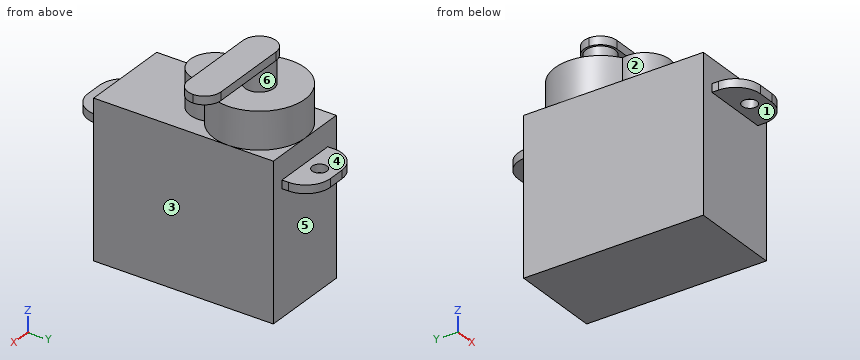
from build123d import *

# Parameters (mm, degrees)
F0_W      = 11
F0_H      = 21.8
F1_DEPTH  = 18.8
F3_W      = 8
F3_H      = 3.8
F3_R      = 0.9
F4_DEPTH  = 1
F6_DEPTH  = 4.5
F7_R      = 1.75
F8_DEPTH  = 3.5
F10_W     = 13.6
F10_H     = 4
F11_DEPTH = 1
F12_R     = 1.99999
F13_R     = 3


# Not quite as in the source:
# - a fillet or chamfer is up to 0.001 mm smaller than in the source, because OpenCascade refuses the exact size


with BuildPart() as f1:
    # F0 (on Top) → F1 (new body)
    with BuildSketch(Plane.XY):
        Rectangle(F0_W, F0_H)
    extrude(amount=F1_DEPTH)

    # F3 (on offset) → F4 (join)
    with BuildSketch(Plane.XY.offset(14.9)):
        with Locations((0, 12.8)):
            Rectangle(F3_W, F3_H)
        with Locations((0, 12.7)):
            Circle(F3_R, mode=Mode.SUBTRACT)
        with Locations((0, -12.8)):
            Rectangle(F3_W, F3_H)
        with Locations((0, -12.7)):
            Circle(F3_R, mode=Mode.SUBTRACT)
    extrude(amount=F4_DEPTH)

    # F5 (on face) → F6 (join)
    with BuildSketch(Plane.XY.offset(18.8)):
        with BuildLine():
            ThreePointArc((-2.9092231591, 0.7324074074), (0, -3), (2.9092231591, 0.7324074074))
            ThreePointArc((2.9092231591, 0.7324074074), (0, 10.9), (-2.9092231591, 0.7324074074))
        make_face()
    extrude(amount=F6_DEPTH)

    # F7 (on face) → F8 (join)
    with BuildSketch(Plane.XY.offset(23.3)):
        with Locations((0, 5.4)):
            Circle(F7_R)
    extrude(amount=F8_DEPTH)

    # F10 (on offset) → F11 (join)
    with BuildSketch(Plane(origin=(0, 0, 26.6), x_dir=(1, 0, 0), z_dir=(0, 0, -1))):
        with Locations((4.8, -5.4)):
            Rectangle(F10_W, F10_H)
    extrude(amount=-F11_DEPTH)

    # F12 (radius 2 in the source; OpenCascade refuses exactly that, so slightly less here)
    f12_edges = [f1.edges().sort_by_distance(p)[0] for p in [
        (11.6, 3.4, 27.1),
        (11.6, 7.4, 27.1),
        (-2, 7.4, 27.1),
        (-2, 3.4, 27.1),
    ]]
    fillet(f12_edges, radius=F12_R)

    # F13
    f13_edges = [f1.edges().sort_by_distance(p)[0] for p in [
        (-4, -14.7, 15.4),
        (4, -14.7, 15.4),
        (4, 14.7, 15.4),
        (-4, 14.7, 15.4),
    ]]
    fillet(f13_edges, radius=F13_R)


solid = f1.part
Read the model definition and answer for the solid it produces. Units are mm, in the model's axes. Face numbers are marked on the shaded views. A direction names the side the tool comes from. Round coordinates to 2 decimals unless told otherwise and drop trailing zeros. Write each loop counter-clockwise with the first axis right and the second up, starting at its lowest first coordinate (ties: lowest second). Pieces come first, ordered by that corner, then holes.
Q1. Find section C-C on z = 24.5. Determine the outline of the cut face in (x, y).
Values:
outline: circle Ø3.5 at (0, 5.4)
Q2. The mould has two halves that part along Z. Classify the marked faces 4, 5 and 6: released by +Z, released by -Z, zero draft, split by the parting line, or undercut.
Values:
face 4: released by +Z
face 5: zero draft
face 6: undercut
Q3. Find section D-D on y = -12.7. Determine the outline of the cut face in (x, z).
Values:
outline: (-3.83, 14.9) - (-0.9, 14.9) - (-0.9, 15.9) - (-3.83, 15.9) - close; (0.9, 14.9) - (3.83, 14.9) - (3.83, 15.9) - (0.9, 15.9) - close
Q4. Find section B-B on y = 0. Determine the outline of the cut face in (x, z).
Values:
outline: (-5.5, 0) - (5.5, 0) - (5.5, 18.8) - (3, 18.8) - (3, 23.3) - (-3, 23.3) - (-3, 18.8) - (-5.5, 18.8) - close
Q5. Straight lines are drawn through the part: line 1 (Y direction, x = 0, z = 15.25); line 2 (Z direction, x = -0.25, y = 3.5); line 3 (Z direction, x = -4.5, y = 7.5). For each, find the intervals that lie inside material, in ascending order.
Values:
line 1: y = -14.7 to -13.6, -11.8 to 11.8, 13.6 to 14.7
line 2: z = 0 to 23.3, 26.6 to 27.6
line 3: z = 0 to 23.3
Q6. A tool of negligible diameter and unlimited length cuts with its end or side. For the marked faces 1, 2 and 3, from which of +Z, -Z, +X, -X, +Y, -Y can it reach the whole face along a straight path? Write none if from no direction.
Values:
face 1: -Z, +X, -X, -Y
face 2: +Z
face 3: -Z, +X, +Y, -Y
Q7. Find section A-A on x = 2.5. Determine the outline of the cut face in (y, z), and give its area (3 significant figures).
Values:
outline: (-14.3, 14.9) - (-10.9, 14.9) - (-10.9, 0) - (10.9, 0) - (10.9, 14.9) - (14.3, 14.9) - (14.3, 15.9) - (10.9, 15.9) - (10.9, 18.8) - (10.3, 18.8) - (10.3, 23.3) - (-1.66, 23.3) - (-1.66, 18.8) - (-10.9, 18.8) - (-10.9, 15.9) - (-14.3, 15.9) - close; (3.4, 26.6) - (7.4, 26.6) - (7.4, 27.6) - (3.4, 27.6) - close
area: 474 mm2
Q8. Flat-ended cylindrical pins translate along their axes: P1, Ø3, axis at x = 1.5, y = -12.5, coming from the +Z side; P2, Ø8, axis at x = 9, y = -2.5, coming from the +Z side; P3, Ø3, axis at x = 2.5, y = 5.5, coming from the -Z side; P4, Ø1.1, axis at x = 0, y = -12.7, coming from the +Z side. Find the tip coordinate at first contact, or state that the pin passes through.
Values:
P1: stops at z = 15.9
P2: stops at z = 18.8
P3: stops at z = 0
P4: passes through
